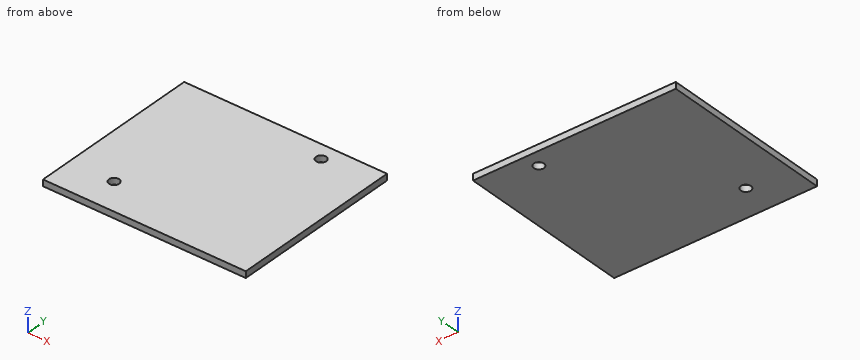
Autodesk Inventor part; units mm, degrees
ref_plane "YZ Plane" through (0, 0, 0) normal (1, 0, 0) x (0, 1, 0)
ref_plane "XZ Plane" through (0, 0, 0) normal (0, 1, 0) x (-1, 0, 0)
ref_plane "XY Plane" through (0, 0, 0) normal (0, 0, 1) x (1, 0, 0)
sketch "Skizze1" plane through (0, 0, 0) normal (0, 0, 1) x (1, 0, 0)
  line L0 (0, 0) -> (63.5, 0)
  line L1 (63.5, 0) -> (63.5, 54.6)
  line L2 (63.5, 54.6) -> (0, 54.6)
  line L3 (0, 54.6) -> (0, 0)
  circle A0 centre (14, 10.2) radius 1.6
  circle A1 centre (47, 49.5) radius 1.6
  dimension "d0" = 54.6
  dimension "d1" = 63.5
  dimension "d2" = 3.2
  dimension "d3" = 3.2
  dimension "d4" = 14
  dimension "d5" = 10.2
  dimension "d6" = 49.5
  dimension "d7" = 47
  dimension "d10" = 33
  dimension "d11" = 39.3
extrude "Extrusion1" add sketch "Skizze1" along normal blind 2
properties part number "SMD_Platine"
Input: part model. Units: mm. Frame: model coordinates. Coordinates: 2 decimals unless noted, no trailing zeros. Order: outer loops, then holes, each group sorted by start corner. A loop starts at its lowest first (then second) coordinate and runs counter-clockwise, first axis right, second up. Notation, with made-up numbers: M -21.5,28.25 L -8.5,28.25 A20 ccw -8.5,42.25 Z; hole C 38.25,62 d4. An arc over 180 degrees is marked long. Answer as CSV lines item,"result".
1. Material intervals for line 1 (Y direction, x = 14, z = 0.4); line 2 (Y direction, x = 47, z = 1.05); line 3 (X direction, y = 48.5, z = 0.9), sorted ascending. Write a range as from..to.
Reported:
line 1,"0..8.6, 11.8..54.6"
line 2,"0..47.9, 51.1..54.6"
line 3,"0..45.75, 48.25..63.5"
2. Section B-B (x = 47). Return the cut outline in (y, z).
Reported:
outline,"M 0,0 L 47.9,0 L 47.9,2 L 0,2 Z; M 51.1,0 L 54.6,0 L 54.6,2 L 51.1,2 Z"
3. Section A-A (y = 10.2). Return the cut outline in (x, z).
Reported:
outline,"M 0,0 L 12.4,0 L 12.4,2 L 0,2 Z; M 15.6,0 L 63.5,0 L 63.5,2 L 15.6,2 Z"
